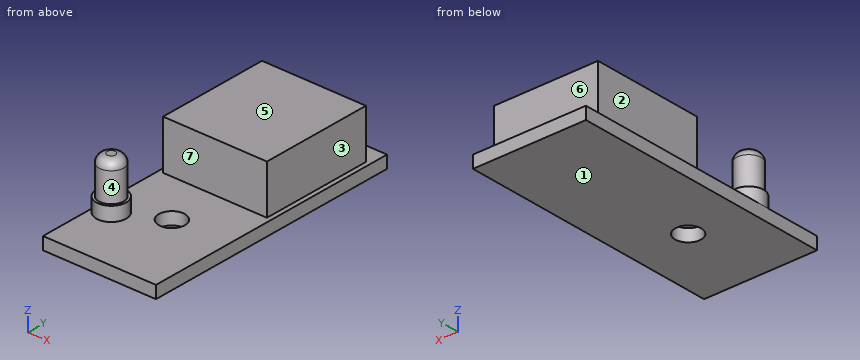
```python
from build123d import *

# Parameters (mm, degrees)
SKETCH1_W           = 13.7
SKETCH1_H           = 32
BOSS_EXTRUDE1_DEPTH = 1.5
SKETCH2_W           = 12.6
SKETCH2_H           = 13.7
BOSS_EXTRUDE2_DEPTH = 5.9
SKETCH3_R           = 1.8
BOSS_EXTRUDE3_DEPTH = 1.7
SKETCH6_R           = 1.5
BOSS_EXTRUDE4_DEPTH = 4.5
FILLET1_R           = 1
SKETCH7_R           = 1.575
CUT_EXTRUDE1_DEPTH  = 2.5


with BuildPart() as part:
    # Sketch1 → Boss-Extrude1 (new body)
    with BuildSketch(Plane.XY):
        Rectangle(SKETCH1_W, SKETCH1_H)
    extrude(amount=BOSS_EXTRUDE1_DEPTH)

    # Sketch2 → Boss-Extrude2 (add)
    with BuildSketch(Plane.XY.offset(1.5)):
        with Locations((0, 6.85)):
            Rectangle(SKETCH2_W, SKETCH2_H)
    extrude(amount=BOSS_EXTRUDE2_DEPTH)

    # Sketch3 → Boss-Extrude3 (add)
    with BuildSketch(Plane.XY.offset(1.5)):
        with Locations((-5.05, -8.6)):
            Circle(SKETCH3_R)
    extrude(amount=BOSS_EXTRUDE3_DEPTH)

    # Sketch6 → Boss-Extrude4 (add)
    with BuildSketch(Plane.XY.offset(3.2)):
        with Locations((-5.05, -8.6)):
            Circle(SKETCH6_R)
    extrude(amount=BOSS_EXTRUDE4_DEPTH)

    # Fillet1
    fillet1_edges = [part.edges().sort_by_distance(p)[0] for p in [
        (-6.55, -8.6, 7.7),
    ]]
    fillet(fillet1_edges, radius=FILLET1_R)

    # Sketch7 → Cut-Extrude1 (cut, through all)
    with BuildSketch(Plane.XY.offset(1.5)):
        with Locations((0, -5.975)):
            Circle(SKETCH7_R)
    extrude(amount=-CUT_EXTRUDE1_DEPTH, mode=Mode.SUBTRACT)


solid = part.part
```
Input: part model. Units: mm. Frame: model coordinates. Face numbers are marked on the shaded views. A direction names the side the tool comes from. Coordinates: 2 decimals unless noted, no trailing zeros. Loops run counter-clockwise (first coordinate to the right, second up) from the corner with the lowest first, then second, coordinate; pieces in that order, holes last.
Q1. Line query: line 1 along Y through (x, z) = (0, 0.7); line 2 along Y through (x, z) = (3.5, 3.25); line 3 along Z through (x, y) = (-6, 13). Output: solid intervals per line, ascending.
Results are:
line 1: y = -16 to -7.55, -4.4 to 16
line 2: y = 0 to 13.7
line 3: z = 0 to 7.4
Q2. Contact query for flat-ended pins moving along their axis: pin 1 (1.5 mm diameter, centred on x = -1, y = 3, fed in from -Z); pin 2 (1.8 mm diameter, centred on y = 8, z = 5, fed in from +X); pin 3 (3 mm diameter, centred on x = 5, z = 4.5, fed in from +Y); pin 4 (1.8 mm diameter, centred on y = 9, z = 4, fed in from -X). Output: stop coordinate, or through.
Results are:
pin 1: stops at z = 0
pin 2: stops at x = 6.3
pin 3: stops at y = 13.7
pin 4: stops at x = -6.3
Q3. Section C-C, the plane y = 1. Return the cut outline in (x, z).
Results are:
outline: (-6.85, 0) - (6.85, 0) - (6.85, 1.5) - (6.3, 1.5) - (6.3, 7.4) - (-6.3, 7.4) - (-6.3, 1.5) - (-6.85, 1.5) - close
Q4. Set-up query: the marked faces 1, 2, 3 and 4. Return all of +Z, -Z, +X, -X, +Y, -Y with unobstructed straight access to the full face (end or side cutting, diameter ignored); none if empty.
Results are:
face 1: -Z, +X, -X, +Y, -Y
face 2: +Z, -X, +Y
face 3: +Z, +X, +Y, -Y
face 4: +Z
Q5. Mould query, pull axis Y, two halves, no side actions, for the marked faces 5, 6 and 7. Classes: +Y half, -Y half, draft (parallel to the pull), parting line (faces both ways), or undercut.
Results are:
face 5: draft
face 6: +Y half
face 7: undercut
Q6. Section A-A, the plane z = 5.25. Return the cut outline in (x, y), and give its area (3 significant figures).
Results are:
outline: circle Ø3 at (-5.05, -8.6); (-6.3, 0) - (6.3, 0) - (6.3, 13.7) - (-6.3, 13.7) - close
area: 180 mm2
Q7. Section B-B, the plane x = 0. Return the cut outline in (y, z).
Results are:
outline: (-16, 0) - (-7.55, 0) - (-7.55, 1.5) - (-16, 1.5) - close; (-4.4, 0) - (16, 0) - (16, 1.5) - (13.7, 1.5) - (13.7, 7.4) - (0, 7.4) - (0, 1.5) - (-4.4, 1.5) - close
Q8. Section D-D, the plane x = 5.5. Return the cut outline in (y, z).
Results are:
outline: (-16, 0) - (16, 0) - (16, 1.5) - (13.7, 1.5) - (13.7, 7.4) - (0, 7.4) - (0, 1.5) - (-16, 1.5) - close
